from build123d import *

# Parameters (mm, degrees)
MODEL_R             = 1.4605
MODEL_R_2           = 2
BOSS_EXTRUDE1_DEPTH = 2.413
SKETCH1_W           = 10
SKETCH1_H           = 24
CUT_EXTRUDE1_DEPTH  = 10


with BuildPart() as part:
    # Model → Boss-Extrude1 (new body, symmetric)
    with BuildSketch(Plane.XY):
        with BuildLine():
            Line((-293.081304326, -31.2683), (-261.331304326, -12.937428953))
            Line((-261.331304326, -12.937428953), (-261.331304326, -5.149171047))
            Line((-261.331304326, -5.149171047), (-293.081304326, 13.1817))
            Line((-293.081304326, 13.1817), (-293.081304326, 51.2817))
            Line((-293.081304326, 51.2817), (-261.331304326, 69.612571047))
            Line((-261.331304326, 69.612571047), (-261.331304326, 76.6817))
            Line((-261.331304326, 76.6817), (-293.081304326, 108.4317))
            Line((-293.081304326, 108.4317), (-293.081304326, 127.4817))
            ThreePointArc((-293.081304326, 127.4817), (-291.221432386, 131.971828061), (-286.731304326, 133.8317))
            Line((-286.731304326, 133.8317), (-267.681304326, 133.8317))
            Line((-267.681304326, 133.8317), (-229.581304326, 95.7317))
            Line((-229.581304326, 95.7317), (-21.581304326, 95.7317))
            Line((-21.581304326, 95.7317), (16.518695674, 133.8317))
            Line((16.518695674, 133.8317), (35.568695674, 133.8317))
            ThreePointArc((35.568695674, 133.8317), (40.058823735, 131.971828061), (41.918695674, 127.4817))
            Line((41.918695674, 127.4817), (41.918695674, 108.4317))
            Line((41.918695674, 108.4317), (10.168695674, 76.6817))
            Line((10.168695674, 76.6817), (10.168695674, 69.612571047))
            Line((10.168695674, 69.612571047), (41.918695674, 51.2817))
            Line((41.918695674, 51.2817), (41.918695674, 13.1817))
            Line((41.918695674, 13.1817), (10.168695674, -5.149171047))
            Line((10.168695674, -5.149171047), (10.168695674, -12.937428953))
            Line((10.168695674, -12.937428953), (41.918695674, -31.2683))
            Line((41.918695674, -31.2683), (41.918695674, -59.836710662))
            Line((41.918695674, -59.836710662), (12.864640386, -80.18057919))
            Line((12.864640386, -80.18057919), (10.168695674, -82.0683))
            Line((10.168695674, -82.0683), (10.168695674, -144.0183))
            Line((10.168695674, -144.0183), (41.918695674, -175.7683))
            Line((41.918695674, -175.7683), (41.918695674, -194.8183))
            ThreePointArc((41.918695674, -194.8183), (40.058823735, -199.308428061), (35.568695674, -201.1683))
            Line((35.568695674, -201.1683), (16.518695674, -201.1683))
            Line((16.518695674, -201.1683), (-26.381304326, -158.2683))
            Line((-26.381304326, -158.2683), (-224.781304326, -158.2683))
            Line((-224.781304326, -158.2683), (-267.681304326, -201.1683))
            Line((-267.681304326, -201.1683), (-286.731304326, -201.1683))
            ThreePointArc((-286.731304326, -201.1683), (-291.221432386, -199.308428061), (-293.081304326, -194.8183))
            Line((-293.081304326, -194.8183), (-293.081304326, -175.7683))
            Line((-293.081304326, -175.7683), (-261.331304326, -144.0183))
            Line((-261.331304326, -144.0183), (-261.331304326, -82.0683))
            Line((-261.331304326, -82.0683), (-293.081304326, -50.3183))
            Line((-293.081304326, -50.3183), (-293.081304326, -31.2683))
        make_face()
        with Locations((-289.525304326, -190.6025)):
            Circle(MODEL_R, mode=Mode.SUBTRACT)
        with Locations((31.352895674, -190.6025)):
            Circle(MODEL_R, mode=Mode.SUBTRACT)
        with Locations((31.352895674, 130.2757)):
            Circle(MODEL_R, mode=Mode.SUBTRACT)
        with Locations((-289.525304326, 130.2757)):
            Circle(MODEL_R, mode=Mode.SUBTRACT)
        with Locations((-277.081304256, -45.4288)):
            Circle(MODEL_R, mode=Mode.SUBTRACT)
        with Locations((-257.081304256, -45.4288)):
            Circle(MODEL_R, mode=Mode.SUBTRACT)
        with Locations((25.918695604, -45.4288)):
            Circle(MODEL_R, mode=Mode.SUBTRACT)
        with Locations((5.918695604, -45.4288)):
            Circle(MODEL_R, mode=Mode.SUBTRACT)
        with Locations((25.918695604, 30.5682)):
            Circle(MODEL_R, mode=Mode.SUBTRACT)
        with Locations((5.918695604, 30.5682)):
            Circle(MODEL_R, mode=Mode.SUBTRACT)
        with Locations((-257.081304256, 30.5682)):
            Circle(MODEL_R, mode=Mode.SUBTRACT)
        with Locations((-277.081304256, 30.5682)):
            Circle(MODEL_R, mode=Mode.SUBTRACT)
        with Locations((-125.581304326, -12.2183)):
            Circle(MODEL_R_2, mode=Mode.SUBTRACT)
        with Locations((-125.581304326, -50.3183)):
            Circle(MODEL_R_2, mode=Mode.SUBTRACT)
        Polygon((-30.331304326, -145.5683), (-68.431304326, -107.4683), (-182.731304326, -107.4683), (-220.831304326, -145.5683), align=None, mode=Mode.SUBTRACT)
        Polygon((-220.831304326, 83.0317), (-182.731304326, 44.9317), (-68.431304326, 44.9317), (-30.331304326, 83.0317), align=None, mode=Mode.SUBTRACT)
        Polygon((-201.781304326, -69.3683), (-233.531304326, -37.6183), (-233.531304326, -24.9183), (-201.781304326, 6.8317), (-182.731304326, 6.8317), (-150.981304326, -24.9183), (-150.981304326, -37.6183), (-182.731304326, -69.3683), align=None, mode=Mode.SUBTRACT)
        Polygon((-100.181304326, -37.6183), (-100.181304326, -24.9183), (-68.431304326, 6.8317), (-49.381304326, 6.8317), (-17.631304326, -24.9183), (-17.631304326, -37.6183), (-49.381304326, -69.3683), (-68.431304326, -69.3683), align=None, mode=Mode.SUBTRACT)
    extrude(amount=BOSS_EXTRUDE1_DEPTH, both=True)

    # Sketch1 → Cut-Extrude1 (cut)
    with BuildSketch(Plane.XY.offset(2.413)):
        with Locations((-267.081304256, -45.4288)):
            Rectangle(SKETCH1_W, SKETCH1_H)
        with Locations((-267.081304256, 30.5712)):
            Rectangle(SKETCH1_W, SKETCH1_H)
        with Locations((15.918695604, 30.5712)):
            Rectangle(SKETCH1_W, SKETCH1_H)
        with Locations((15.918695604, -45.4288)):
            Rectangle(SKETCH1_W, SKETCH1_H)
    extrude(amount=-CUT_EXTRUDE1_DEPTH, mode=Mode.SUBTRACT)


solid = part.part
Design review of the part built by this model. Coordinates are the model's own, in mm. A direction names the side the tool comes from. Round coordinates to 2 decimals unless told otherwise and drop trailing zeros. Write each loop counter-clockwise with the first axis right and the second up, starting at its lowest first coordinate (ties: lowest second). Pieces come first, ordered by that corner, then holes. Notation, with made-up numbers: (40, -37) - (94, -37) arc R20 ccw to (94, -3) - close; hole circle Ø4 at (21.5, -38). An arc over 180 degrees is marked (long way). Return JSON: item names as keys, results as strings. Group by question number.
Item 1: Machinability: for faces 4 (the face through (-245.931, -179.418, 0.034)), 5 (the face through (25.821, 60.575, 0.034)), 6 (the face through (-248.9, 115.05, 0.03)), which of the approach directions +Z, -Z, +X, -X, +Y, -Y give a long, thin tool a straight path to every point of the face, cutting with its end or side? Answer none if there is none.
Item 2: We need section C-C on x = -158. Write out the cut boundary in (y, z).
Item 3: The part is to be moulded in two halves that separate along X. For faces 1 (the face through (-49.1, -126.8, 0)), 2 (the face through (-276.98, 92.33, 0.03)), 3 (the face through (-123, -31, 2.413)), say which applies: pulls with the +X half, pulls with the -X half, needs draft (parallel to the pull), parting line crosses it, or undercut.
Item 4: We need section A-A on x = -80. Write out the cut boundary in (y, z), and give its area (3 significant figures).
Item 5: Insertion check: P1, Ø1.4, axis at x = -130, z = -1, coming from the -Y side; P2, Ø1, axis at x = -258, z = 0, coming from the +Y side; P3, Ø2.5, axis at x = -120, z = 1, coming from the +Y side; P4, Ø12, axis at x = -126.5, y = 73, coming from the -Z side. Each pin has a flat end and moves straight along its axis. Give the tip position at first contact, or say it passes through.
Item 6: We need section D-D on z = -0.95. Give the number of separate pieces and of enclosed holes in the cut face, and give its area (3 significant figures).
Item 7: For probe 1 along Y at (x, z) = (-134, -1.95); probe 2 along Y at (x, z) = (-89.5, 2.2); probe 3 along X at (y, z) = (-41.5, -2.05), list the stretches that pass through material, from the lowest coordinate up. Write a range as [from, to].
Item 8: We need section B-B on y = -166. Write out the cut boundary in (x, z).
Model answer:
{
 "1": {"face 4": "+Z, -Z, -Y", "face 5": "+Z, -Z, +X", "face 6": "+Z, -Z, +Y"},
 "2": {"outline": "(-158.27, -2.41) - (-145.57, -2.41) - (-145.57, 2.41) - (-158.27, 2.41) - close; (-107.47, -2.41) - (-44.64, -2.41) - (-44.64, 2.41) - (-107.47, 2.41) - close; (-17.9, -2.41) - (44.93, -2.41) - (44.93, 2.41) - (-17.9, 2.41) - close; (83.03, -2.41) - (95.73, -2.41) - (95.73, 2.41) - (83.03, 2.41) - close"},
 "3": {"face 1": "undercut", "face 2": "pulls with the -X half", "face 3": "needs draft"},
 "4": {"outline": "(-158.27, -2.41) - (-145.57, -2.41) - (-145.57, 2.41) - (-158.27, 2.41) - close; (-107.47, -2.41) - (-57.8, -2.41) - (-57.8, 2.41) - (-107.47, 2.41) - close; (-4.74, -2.41) - (44.93, -2.41) - (44.93, 2.41) - (-4.74, 2.41) - close; (83.03, -2.41) - (95.73, -2.41) - (95.73, 2.41) - (83.03, 2.41) - close", "area": "602 mm²"},
 "5": {"P1": "stops at y = -158.27", "P2": "stops at y = 124.65", "P3": "stops at y = 95.73", "P4": "passes through"},
 "6": {"separate pieces": "1", "enclosed holes": "22", "area": "61,700 mm²"},
 "7": {"probe 1": "y = [-158.27, -145.57], [-107.47, 44.93], [83.03, 95.73]", "probe 2": "y = [-158.27, -145.57], [-107.47, -48.3], [-14.24, 44.93], [83.03, 95.73]", "probe 3": "x = [-293.08, -272.08], [-262.08, -229.65], [-154.86, -96.3], [-21.51, 10.92], [20.92, 41.92]"},
 "8": {"outline": "(-283.31, -2.41) - (-232.51, -2.41) - (-232.51, 2.41) - (-283.31, 2.41) - close; (-18.65, -2.41) - (32.15, -2.41) - (32.15, 2.41) - (-18.65, 2.41) - close"}
}
